Here's how the part is built. I have some questions about the finished solid (model axes, mm). A direction names the side the tool comes from. Coordinates: 2 decimals unless noted, no trailing zeros. Loops run counter-clockwise (first coordinate to the right, second up) from the corner with the lowest first, then second, coordinate; pieces in that order, holes last. Notation, with made-up numbers: M 28,71 L 61,71 A19 ccw 61,99 Z; hole C 3,-19 d11. An arc over 180 degrees is marked long. Use one line per item in the form item = value. Start each with the question number.
(1) Imagine slicing it at A-A, the plane y = 28.9. Please give me the cut outline in (x, z).
(2) Please list where these lines run through material, in increasing order: L1, parallel to X at y = 15, z = 2; L2, parallel to Y at x = 7.5, z = 6.5; L3, parallel to X at y = 8, z = 44.
(3) Imagine slicing it at D-D, the plane y = 40. Please give me the cut outline in (x, z), and give its area (3 significant figures).
(4) Thinking about a two-plate mould opening in Y: for faces 1 (the flat face through (8.5, 53, 43)), 2 (the cylindrical face through (4, 4, 9)), 3 (the cylindrical face through (4.191, 3.874, 72.398)), which applies, +Y half, -Y half, draft (parallel to the pull), parting line (faces both ways), or undercut?
(5) On a 3-axis mill with a long thin cutter (end or side, diameter ignored), from which of +Z, -Z, +X, -X, +Y, -Y can I reach the whole of each face in a straight line? I mean faces 4 (the cylindrical face through (4.31, 28.82, 4.75)), 5 (the cylindrical face through (5, 16.2, 3)), 6 (the cylindrical face through (4.19, 54.36, 72.96)), 7 (the flat face through (5, 7.5, 43)), 8 (the flat face through (4, 4.5, 44)). Say none if no direction works.
(6) Imagine slicing it at B-B, the plane z = 44. State how many separate pieces and enclosed holes the cut face has, and give its area (3 significant figures).
(7) Will these pins go through, and if not, where does the flat tip stop? P1, Ø0.9, axis at y = 35.5, z = 49, coming from the +X side; P2, Ø3, axis at x = 5.5, z = 47, coming from the -Y side; P3, Ø3, axis at x = 5, z = 55, coming from the +Y side.
```python
from build123d import *

# Parameters (mm, degrees)
BOSS_EXTRUDE1_DEPTH            = 86.5
M3X0_5_TAPPED_HOLE2_AT_2_COUNT = 2
M3X0_5_TAPPED_HOLE2_AT_2_PITCH = 27.4
M3X0_5_TAPPED_HOLE1_D          = 2.5
SKETCH14_R                     = 3.5
CUT_EXTRUDE3_DEPTH             = 9.5
CUT_EXTRUDE1_DEPTH             = 9.5
SKETCH15_W                     = 62
SKETCH15_H                     = 7.5
CUT_EXTRUDE4_DEPTH             = 9.5
SKETCH16_W                     = 62
SKETCH16_H                     = 4.5
CUT_EXTRUDE5_DEPTH             = 9.5
FILLET2_R                      = 4
FILLET3_R                      = 4


with BuildPart() as part:
    # Sketch1 → Boss-Extrude1 (new body)
    with BuildSketch(Plane.XY):
        Polygon((0, 0), (0, 60.8), (8.5, 60.8), (8.5, 50.3), (2.4, 50.3), (2.4, 48.6), (8.5, 48.6), (8.5, 36.6), (2.5, 36.6), (2.5, 34.9), (8.5, 34.9), (8.5, 22.9), (2.5, 22.9), (2.5, 21.2), (8.5, 21.2), (8.5, 9.2), (2.5, 9.2), (2.5, 7.5), (8.5, 7.5), (8.5, 0), align=None)
    extrude(amount=BOSS_EXTRUDE1_DEPTH)

    # Sketch4 → M3x0.5 Tapped Hole2 (revolve, cut)
    with BuildSketch(Plane(origin=(4.25, 42.6, 86.5), x_dir=(0, -1, 0), z_dir=(1, 0, 0))):
        Polygon((0, 0), (0, 6.751075774), (1.25, 6), (1.25, 0), align=None)
    m3x0_5_tapped_hole2 = revolve(axis=Axis((4.25, 42.6, 92.85), (0, 0, -1)), mode=Mode.SUBTRACT)

    # M3x0.5 Tapped Hole2 at 2: M3x0.5 Tapped Hole2 ×2
    with Locations(*[(0, -i * M3X0_5_TAPPED_HOLE2_AT_2_PITCH, 0) for i in range(1, M3X0_5_TAPPED_HOLE2_AT_2_COUNT)]):
        add(m3x0_5_tapped_hole2, mode=Mode.SUBTRACT)

    # Mirror1: M3x0.5 Tapped Hole2 across plane
    add(m3x0_5_tapped_hole2.mirror(Plane.XY.offset(43.25)), mode=Mode.SUBTRACT)

    # Mirror1 copy 1 sketch → Mirror1 copy 1 (revolve, cut)
    with BuildSketch(Plane(origin=(4.25, 15.2, 0), x_dir=(0, -1, 0), z_dir=(1, 0, 0))):
        Polygon((0, 0), (0, -6.751075774), (1.25, -6), (1.25, 0), align=None)
    revolve(axis=Axis((4.25, 15.2, -6.35), (0, 0, -1)), mode=Mode.SUBTRACT)

    # M3x0.5 Tapped Hole1 (through all)
    with Locations(Plane.ZY):
        with Locations((8.25, 5), (8.25, 54)):
            m3x0_5_tapped_hole1 = Hole(M3X0_5_TAPPED_HOLE1_D / 2)

    # Mirror2: M3x0.5 Tapped Hole1 across plane
    add(m3x0_5_tapped_hole1.mirror(Plane(origin=(0, 0, 43.25), x_dir=(1, 0, 0), z_dir=(0, 0, -1))), mode=Mode.SUBTRACT)

    # Sketch14 → Cut-Extrude3 (cut, through all)
    with BuildSketch(Plane(origin=(8.5, 0, 0), x_dir=(0, 0, -1), z_dir=(1, 0, 0))):
        with BuildLine():
            Line((-8.25, 32.4), (-78.25, 32.4))
            ThreePointArc((-78.25, 32.4), (-75.775126266, 31.374873734), (-74.75, 28.9))
            ThreePointArc((-74.75, 28.9), (-75.775126266, 26.425126266), (-78.25, 25.4))
            Line((-78.25, 25.4), (-8.25, 25.4))
            ThreePointArc((-8.25, 25.4), (-11.75, 28.9), (-8.25, 32.4))
        make_face()
        with Locations((-78.25, 28.9)):
            Circle(SKETCH14_R)
        with Locations((-8.25, 28.9)):
            Circle(SKETCH14_R)
    extrude(amount=-CUT_EXTRUDE3_DEPTH, mode=Mode.SUBTRACT)

    # Sketch12 → Cut-Extrude1 (cut, through all)
    with BuildSketch(Plane(origin=(8.5, 0, 0), x_dir=(0, 0, -1), z_dir=(1, 0, 0))):
        with BuildLine():
            Line((-14.75, 46.1), (-71.75, 46.1))
            ThreePointArc((-71.75, 46.1), (-75.25, 42.6), (-71.75, 39.1))
            Line((-71.75, 39.1), (-14.75, 39.1))
            ThreePointArc((-14.75, 39.1), (-11.25, 42.6), (-14.75, 46.1))
        make_face()
        with BuildLine():
            Line((-14.75, 18.7), (-71.75, 18.7))
            ThreePointArc((-71.75, 18.7), (-75.25, 15.2), (-71.75, 11.7))
            Line((-71.75, 11.7), (-14.75, 11.7))
            ThreePointArc((-14.75, 11.7), (-11.25, 15.2), (-14.75, 18.7))
        make_face()
    extrude(amount=-CUT_EXTRUDE1_DEPTH, mode=Mode.SUBTRACT)

    # Sketch15 → Cut-Extrude4 (cut, through all)
    with BuildSketch(Plane(origin=(8.5, 0, 0), x_dir=(0, 0, -1), z_dir=(1, 0, 0))):
        with Locations((-43.25, 57.05)):
            Rectangle(SKETCH15_W, SKETCH15_H)
    extrude(amount=-CUT_EXTRUDE4_DEPTH, mode=Mode.SUBTRACT)

    # Sketch16 → Cut-Extrude5 (cut, through all)
    with BuildSketch(Plane(origin=(8.5, 0, 0), x_dir=(0, 0, -1), z_dir=(1, 0, 0))):
        with Locations((-43.25, 2.25)):
            Rectangle(SKETCH16_W, SKETCH16_H)
    extrude(amount=-CUT_EXTRUDE5_DEPTH, mode=Mode.SUBTRACT)

    # Fillet2
    fillet2_edges = [part.edges().sort_by_distance(p)[0] for p in [
        (4.25, 53.3, 12.25),
        (4.25, 53.3, 74.25),
        (4.25, 4.5, 12.25),
        (4.25, 4.5, 74.25),
    ]]
    fillet(fillet2_edges, radius=FILLET2_R)

    # Fillet3
    fillet3_edges = [part.edges().sort_by_distance(p)[0] for p in [
        (4.25, 0, 12.25),
        (4.25, 0, 74.25),
        (4.25, 60.8, 12.25),
        (4.25, 60.8, 74.25),
    ]]
    fillet(fillet3_edges, radius=FILLET3_R)


solid = part.part
```
Answer:
q1.outline = M 0,0 L 8.5,0 L 8.5,4.75 L 0,4.75 Z; M 0,81.75 L 8.5,81.75 L 8.5,86.5 L 0,86.5 Z
q2.L1 = 0 to 3.02, 5.48 to 8.5
q2.L2 = 0 to 7.5, 9.2 to 21.2, 22.9 to 25.87, 31.93 to 34.9, 36.6 to 48.6, 50.3 to 60.8
q2.L3 = 0 to 2.5
q3.outline = M 0,0 L 8.5,0 L 8.5,12.41 L 0,12.41 Z; M 0,74.09 L 8.5,74.09 L 8.5,86.5 L 0,86.5 Z
q3.area = 211 mm²
q4.face_1 = draft
q4.face_2 = undercut
q4.face_3 = -Y half
q5.face_4 = +X, -X
q5.face_5 = -Z
q5.face_6 = +X, -X, +Y
q5.face_7 = +Z, -Z, +X
q5.face_8 = +X, -X, -Y
q6.separate_pieces = 4
q6.enclosed_holes = 0
q6.area = 195 mm²
q7.P1 = 2.5
q7.P2 = 4.5
q7.P3 = 53.3
